Input: part model. Units: mm. Frame: model coordinates. Face numbers are marked on the shaded views. A direction names the side the tool comes from. Coordinates: 2 decimals unless noted, no trailing zeros. Order: outer loops, then holes, each group sorted by start corner. A loop starts at its lowest first (then second) coordinate and runs counter-clockwise, first axis right, second up. Notation, with made-up numbers: (69, 79) -> (126, 79) arc R16 ccw to (126, 97) -> close; hole circle Ø1 at (-24.75, 74). An arc over 180 degrees is marked (long way). Use one line per item in the form item = value. Start each with the question number.
1) Section query D-D on z = -28. Output: boundary loops of the cut face in (x, y).
2) Section query B-B on x = -5. Output: boundary loops of the cut face in (y, z).
3) Section query C-C on y = 1.5. Output: boundary loops of the cut face in (x, z).
4) Pin query (flat end, axial travel): pin 1 (12 mm diameter, centred on x = -3.5, z = -17, fed in from +Y); pin 2 (10 mm diameter, centred on y = 14.5, z = -22, fed in from +X); pin 3 (8 mm diameter, centred on y = 15, z = -17.5, fed in from +X); pin 4 (13 mm diameter, centred on x = -1.5, z = 0, fed in from +Y). Return the tip coordinate at first contact, or that it passes through.
5) Draft query along X for the marked faces 1, 2 and 3. Return one class per face: pulls with the +X half, pulls with the -X half, needs draft (parallel to the pull), parting line crosses it, or undercut.
6) Ray query, line 1 along Y through (x, z) = (0, -23); line 2 along X through (y, z) = (0, 3.5). Return the intervals inside material, ascending.
7) Section query A-A on z = 0. Output: boundary loops of the cut face in (x, y), then the cut area to 3 significant figures.
8) Access query for the marked faces 4 and 5. Directions: +Z, -Z, +X, -X, +Y, -Y. A direction counts if a zero-diameter tool reaches every point of the face in a straight line with its end or side. Return the directions, or none.
from build123d import *

# Parameters (mm, degrees)
SKETCH1_W          = 16.66875
SKETCH1_H          = 68.2625
SKETCH2_W          = 16.66875
SKETCH2_H          = 34.13125
SKETCH7_R          = 12.7
CUT_EXTRUDE1_DEPTH = 69.2625
CUT_EXTRUDE2_REACH = 52.8
SKETCH8_R          = 12.7
SKETCH9_R          = 13.096875
CUT_EXTRUDE3_DEPTH = 19.05
SKETCH10_R         = 13.096875
CUT_EXTRUDE4_DEPTH = 19.05
SKETCH11_R         = 13.096875
CUT_EXTRUDE5_DEPTH = 19.05


with BuildPart() as part:
    # Sketch1 → Revolve1 (revolve)
    with BuildSketch(Plane(origin=(0, 0, 0), x_dir=(1, 0, 0), z_dir=(0, 1, 0))):
        with Locations((8.334375, 0)):
            Rectangle(SKETCH1_W, SKETCH1_H)
    revolve(axis=Axis((0, 0, 118.243982537), (0, 0, -1)))

    # Sketch2 → Revolve2 (revolve)
    with BuildSketch(Plane.XY):
        with Locations((-8.334375, 17.065625)):
            Rectangle(SKETCH2_W, SKETCH2_H)
    revolve(axis=Axis((0, 0, 0), (0, 1, 0)))

    # Sketch7 → Cut-Extrude1 (cut, through all)
    with BuildSketch(Plane.XY.offset(34.13125)):
        Circle(SKETCH7_R)
    extrude(amount=-CUT_EXTRUDE1_DEPTH, mode=Mode.SUBTRACT)

    # Sketch8 → Cut-Extrude2 (cut, up to next)
    with BuildSketch(Plane(origin=(0, 34.13125, 0), x_dir=(1, 0, 0), z_dir=(0, 1, 0)), mode=Mode.PRIVATE) as cut_extrude2_sk1:
        Circle(SKETCH8_R)
    cut_extrude2_tool1 = extrude(cut_extrude2_sk1.sketch, amount=-CUT_EXTRUDE2_REACH, mode=Mode.PRIVATE) & part.part
    add(cut_extrude2_tool1.solids().sort_by_distance((0, 34.13125, 0))[0], mode=Mode.SUBTRACT)

    # Sketch9 → Cut-Extrude3 (cut)
    with BuildSketch(Plane.XY.offset(34.13125)):
        Circle(SKETCH9_R)
    extrude(amount=-CUT_EXTRUDE3_DEPTH, mode=Mode.SUBTRACT)

    # Sketch10 → Cut-Extrude4 (cut)
    with BuildSketch(Plane(origin=(0, 0, -34.13125), x_dir=(-1, 0, 0), z_dir=(0, 0, -1))):
        Circle(SKETCH10_R)
    extrude(amount=-CUT_EXTRUDE4_DEPTH, mode=Mode.SUBTRACT)

    # Sketch11 → Cut-Extrude5 (cut)
    with BuildSketch(Plane(origin=(0, 34.13125, 0), x_dir=(1, 0, 0), z_dir=(0, 1, 0))):
        Circle(SKETCH11_R)
    extrude(amount=-CUT_EXTRUDE5_DEPTH, mode=Mode.SUBTRACT)


solid = part.part
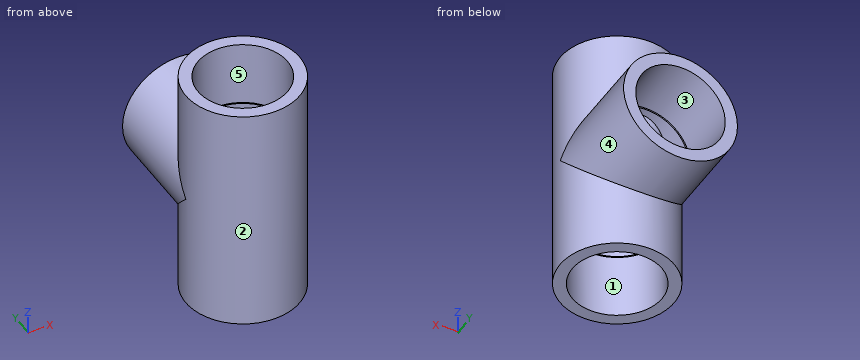
Answers below:
q1.outline = circle Ø33.34 at (0, 0); hole circle Ø26.19 at (0, 0)
q2.outline = (-15.9, -34.13) -> (-12.1, -34.13) -> (-12.1, -15.08) -> (-11.67, -15.08) -> (-11.67, 15.08) -> (-12.1, 15.08) -> (-12.1, 34.13) -> (-15.9, 34.13) -> close; (11.67, -15.08) -> (12.1, -15.08) -> (12.1, -34.13) -> (15.9, -34.13) -> (15.9, -15.9) -> (34.13, -15.9) -> (34.13, -12.1) -> (15.08, -12.1) -> (15.08, -11.67) -> (11.67, -11.67) -> close; (11.67, 11.67) -> (15.08, 11.67) -> (15.08, 12.1) -> (34.13, 12.1) -> (34.13, 15.9) -> (15.9, 15.9) -> (15.9, 34.13) -> (12.1, 34.13) -> (12.1, 15.08) -> (11.67, 15.08) -> close
q3.outline = (-16.6, -34.13) -> (-13.01, -34.13) -> (-13.01, -15.08) -> (-12.61, -15.08) -> (-12.61, -1.5) arc R12.7 cw to (-12.61, 1.5) -> (-12.61, 15.08) -> (-13.01, 15.08) -> (-13.01, 34.13) -> (-16.6, 34.13) -> (-16.6, 1.5) arc R16.67 ccw to (-16.6, -1.5) -> close; (12.61, -15.08) -> (13.01, -15.08) -> (13.01, -34.13) -> (16.6, -34.13) -> (16.6, -1.5) arc R16.67 ccw to (16.6, 1.5) -> (16.6, 34.13) -> (13.01, 34.13) -> (13.01, 15.08) -> (12.61, 15.08) -> (12.61, 1.5) arc R12.7 cw to (12.61, -1.5) -> close
q4.pin_1 = 34.13
q4.pin_2 = 13.7
q4.pin_3 = 12.52
q4.pin_4 = -9.86
q5.face_1 = undercut
q5.face_2 = parting line crosses it
q5.face_3 = undercut
q6.line_1 = -16.67 to -13.1, 13.1 to 16.67
q6.line_2 = -16.67 to -12.7, 12.7 to 16.67
q7.outline = (-16.67, 0) arc R16.67 ccw to (16.67, 0) -> (16.67, 34.13) -> (13.1, 34.13) -> (13.1, 15.08) -> (12.7, 15.08) -> (12.7, 0) arc R12.7 cw to (-12.7, 0) -> (-12.7, 15.08) -> (-13.1, 15.08) -> (-13.1, 34.13) -> (-16.67, 34.13) -> close
q7.area = 439 mm^2
q8.face_4 = +Y
q8.face_5 = +Z
